The model under review builds one solid part; all positions refer to its coordinate system, in mm. A direction names the side the tool comes from. Round coordinates to 2 decimals unless told otherwise and drop trailing zeros. Order: outer loops, then holes, each group sorted by start corner. A loop starts at its lowest first (then second) coordinate and runs counter-clockwise, first axis right, second up. Notation, with made-up numbers: M 55.5,17 L 108.5,17 A19 cw 108.5,28 Z; hole C 20,0 d8. An arc over 180 degrees is marked long. Use a Markdown table: item, result. Add a question column.
1. Consider section A-A on z = 93. State the section outline as (x, y) points.
2. For faces 1 (the flat face through (-71, -24.65, 4)), 2 (the flat face through (-10, 6, 67)), 3 (the flat face through (-132.535, 0.623, -329.663)), list the 3-axis set-ups (+Z, -Z, +X, -X, +Y, -Y) from which the entire face can be reached by the end or side of a thin tool; tool diameter is ignored.
3. Insertion check: P1, Ø6, axis at x = -121.5, z = 306.5, coming from the +Y side; P2, Ø1.5, axis at x = -47, y = 52.5, coming from the -Z side; P3, Ø1.5, axis at x = -87.5, z = -127.5, coming from the +Y side. Each pin has a flat end and moves straight along its axis. Give the tip position at first contact, or say it passes through.
4. Consider section C-C on y = -34.5. State the section outline as (x, z) points, then the cut area to 3 significant figures.
5. To check wall thickness, follow probe 1 along X at (y, z) = (-13, 70.5); probe 2 along Y at (x, z) = (-118.5, 23.5); probe 3 along Z at (x, y) = (-51, -9). State the ranges of each line that lie inside material, in increasing order.
6. Consider section B-B on x = -93. State the section outline as (y, z) points, then the cut area to 3 significant figures.
from build123d import *

# Parameters (mm, degrees)
SKETCH1_W            = 595.899
SKETCH1_H            = 29.3
BOSS_EXTRUDE1_DEPTH  = 10
SKETCH2_W            = 140
SKETCH2_H            = 595.899
BOSS_EXTRUDE2_DEPTH  = 10
SKETCH4_R            = 5
CUT_EXTRUDE1_DEPTH   = 1000
BOSS_EXTRUDE5_DEPTH  = 10
BOSS_EXTRUDE6_DEPTH  = 10
BOSS_EXTRUDE7_REACH  = 759.768
SKETCH9_W            = 120
SKETCH9_H            = 9.145365746
SKETCH18_W           = 120
SKETCH18_H           = 5
CUT_EXTRUDE4_DEPTH   = 595.899
BOSS_EXTRUDE8_DEPTH  = 10
BOSS_EXTRUDE9_DEPTH  = 10
BOSS_EXTRUDE11_DEPTH = 120
SKETCH15_R           = 5
CUT_EXTRUDE2_DEPTH   = 200
SKETCH16_R           = 5
CUT_EXTRUDE3_DEPTH   = 200
CUT_EXTRUDE5_REACH   = 825.564
SKETCH21_W           = 120
SKETCH21_H           = 5
CUT_EXTRUDE6_DEPTH   = 500


with BuildPart() as part:
    # Sketch1 → Boss-Extrude1 (new body)
    with BuildSketch(Plane(origin=(0, 0, 0), x_dir=(0, 0, -1), z_dir=(1, 0, 0))):
        Rectangle(SKETCH1_W, SKETCH1_H)
    boss_extrude1 = extrude(amount=-BOSS_EXTRUDE1_DEPTH)

    # Sketch2 → Boss-Extrude2 (add)
    with BuildSketch(Plane.XZ.offset(14.65)):
        with Locations((-70, 0)):
            Rectangle(SKETCH2_W, SKETCH2_H)
    extrude(amount=BOSS_EXTRUDE2_DEPTH)

    # Mirror2: Boss-Extrude1 across plane
    add(boss_extrude1.mirror(Plane.ZY.offset(70)))

    # Sketch4 → Cut-Extrude1 (cut, symmetric)
    with BuildSketch(Plane.ZY.offset(10)):
        with Locations((-278.7995, 0)):
            Circle(SKETCH4_R)
        with Locations((-193.6995, 0)):
            Circle(SKETCH4_R)
        with Locations((-108.5995, 0)):
            Circle(SKETCH4_R)
        with Locations((-23.4995, 0)):
            Circle(SKETCH4_R)
        with Locations((61.6005, 0)):
            Circle(SKETCH4_R)
        with Locations((146.7005, 0)):
            Circle(SKETCH4_R)
        with Locations((231.8005, 0)):
            Circle(SKETCH4_R)
        with Locations((289.949492565, 0)):
            Circle(SKETCH4_R)
    extrude(amount=CUT_EXTRUDE1_DEPTH, both=True, mode=Mode.SUBTRACT)

    # Sketch7 → Boss-Extrude5 (add)
    with BuildSketch(Plane.ZY.offset(140)):
        Polygon((297.9495, -24.65), (492.560117959, 61.427061861), (478.021751538, 94.296683709), (297.9495, 14.65), align=None)
    extrude(amount=-BOSS_EXTRUDE5_DEPTH)

    # Sketch8 → Boss-Extrude6 (add)
    with BuildSketch(Plane(origin=(0, 0, 0), x_dir=(0, 0, -1), z_dir=(1, 0, 0))):
        Polygon((-297.9495, 14.65), (-478.021751538, 94.296683709), (-492.560117959, 61.427061861), (-297.9495, -24.65), align=None)
    extrude(amount=-BOSS_EXTRUDE6_DEPTH)

    # Boss-Extrude7: up to this face of the body (flat: up to its plane)
    boss_extrude7_end = Plane(part.part.faces().sort_by_distance((-70, -19.65, 297.9495))[0])
    # Sketch9 → Boss-Extrude7 (add, up to the picked face)
    with BuildSketch(Plane(origin=(0, 192.265107265, 434.689922355), x_dir=(1, 0, 0), z_dir=(0, 0.404503218, 0.914536575)), mode=Mode.PRIVATE) as boss_extrude7_sk1:
        with Locations((-70, -138.492175371)):
            Rectangle(SKETCH9_W, SKETCH9_H)
    boss_extrude7_tool1 = split(extrude(boss_extrude7_sk1.sketch, amount=-BOSS_EXTRUDE7_REACH, mode=Mode.PRIVATE), bisect_by=boss_extrude7_end, keep=Keep.BOTH, mode=Mode.PRIVATE)
    add(boss_extrude7_tool1.solids().sort_by_distance((-70, 65.608948, 490.710453))[0])

    # Sketch18 → Cut-Extrude4 (cut)
    with BuildSketch(Plane(origin=(0, 0, -297.9495), x_dir=(-1, 0, 0), z_dir=(0, 0, -1))):
        with Locations((70, -17.15)):
            Rectangle(SKETCH18_W, SKETCH18_H)
    extrude(amount=-CUT_EXTRUDE4_DEPTH, mode=Mode.SUBTRACT)

    # Sketch10 → Boss-Extrude8 (add)
    with BuildSketch(Plane.ZY.offset(140)):
        Polygon((-297.9495, -24.65), (-345.962670166, -45.886418968), (-360.501036587, -13.016797119), (-297.9495, 14.65), align=None)
    extrude(amount=-BOSS_EXTRUDE8_DEPTH)

    # Sketch11 → Boss-Extrude9 (add)
    with BuildSketch(Plane(origin=(0, 0, 0), x_dir=(0, 0, -1), z_dir=(1, 0, 0))):
        Polygon((297.9495, -24.65), (345.962670166, -45.886418968), (360.501036587, -13.016797119), (297.9495, 14.65), align=None)
    extrude(amount=-BOSS_EXTRUDE9_DEPTH)

    # Sketch14 → Boss-Extrude11 (add)
    with BuildSketch(Plane(origin=(-130, 0, 0), x_dir=(0, 0, -1), z_dir=(1, 0, 0))):
        Polygon((297.9495, -24.65), (345.962670166, -45.886418968), (347.812335105, -41.704533236), (297.9495, -19.65), align=None)
    extrude(amount=BOSS_EXTRUDE11_DEPTH)

    # Sketch15 → Cut-Extrude2 (cut)
    with BuildSketch(Plane.ZY.offset(140)):
        with Locations((321.409072715, 8.952548986)):
            Circle(SKETCH15_R)
        with Locations((372.623120892, 31.604729219)):
            Circle(SKETCH15_R)
        with Locations((423.83716907, 54.256909451)):
            Circle(SKETCH15_R)
        with Locations((475.051217247, 76.909089683)):
            Circle(SKETCH15_R)
    extrude(amount=-CUT_EXTRUDE2_DEPTH, mode=Mode.SUBTRACT)

    # Sketch16 → Cut-Extrude3 (cut)
    with BuildSketch(Plane.ZY.offset(140)):
        with Locations((-325.297580118, -10.284676689)):
            Circle(SKETCH16_R)
    extrude(amount=-CUT_EXTRUDE3_DEPTH, mode=Mode.SUBTRACT)

    # Cut-Extrude5: up to this face of the body (flat: up to its plane)
    cut_extrude5_end = Plane(part.part.faces().sort_by_distance((-70, -17.15, 297.9495))[0])
    # Sketch21 → Cut-Extrude5 (cut, up to the picked face)
    with BuildSketch(Plane(origin=(0, 192.265107265, 434.689922355), x_dir=(1, 0, 0), z_dir=(0, 0.404503218, 0.914536575)), mode=Mode.PRIVATE) as cut_extrude5_sk1:
        with Locations((-70, -136.419492498)):
            Rectangle(SKETCH21_W, SKETCH21_H)
    cut_extrude5_tool1 = split(extrude(cut_extrude5_sk1.sketch, amount=-CUT_EXTRUDE5_REACH, mode=Mode.PRIVATE), bisect_by=cut_extrude5_end, keep=Keep.BOTH, mode=Mode.PRIVATE)
    add(cut_extrude5_tool1.solids().sort_by_distance((-70, 67.504492, 489.872046))[0], mode=Mode.SUBTRACT)

    # Sketch23 → Cut-Extrude6 (cut, symmetric)
    with BuildSketch(Plane(origin=(0, 14.65, 0), x_dir=(1, 0, 0), z_dir=(0, 1, 0))):
        Polygon((-140, -297.9495), (-140, 297.9495), (-140, 372.239264408), (-135, 372.239264408), (-135, 297.9495), (-135, -297.9495), (-135, -501.796935229), (-140, -501.796935229), align=None)
    cut_extrude6 = extrude(amount=CUT_EXTRUDE6_DEPTH, both=True, mode=Mode.SUBTRACT)

    # Mirror3: Cut-Extrude6 across plane
    add(cut_extrude6.mirror(Plane.ZY.offset(70)), mode=Mode.SUBTRACT)


solid = part.part
Answer block:
| question | item | result |
|---|---|---|
| 1 | outline | M -135,-24.65 L -5,-24.65 L -5,14.65 L -10,14.65 L -10,-19.65 L -130,-19.65 L -130,14.65 L -135,14.65 Z |
| 2 | face 1 | +Z, +X, -X, -Y |
| 2 | face 2 | -Z, +Y |
| 2 | face 3 | -Z, +X, -X, +Y |
| 3 | P1 | y = -15.01 |
| 3 | P2 | z = 460.43 |
| 3 | P3 | y = -19.65 |
| 4 | outline | M -135,-351 L -130,-351 L -130,-331.52 L -10,-331.52 L -10,-351 L -5,-351 L -5,-320.22 L -135,-320.22 Z |
| 4 | area | 1,660 mm^2 |
| 5 | probe 1 | -135 to -130, -10 to -5 |
| 5 | probe 2 | -24.65 to -19.65 |
| 5 | probe 3 | 323.08 to 333.33 |
| 6 | outline | M -45.89,-345.96 L -41.7,-347.81 L -19.65,-297.95 L -19.65,297.95 L -20.12,297.95 L 65.22,490.88 L 61.43,492.56 L -24.65,297.95 L -24.65,-297.95 Z |
| 6 | area | 4,100 mm^2 |
